Could you check a few things on this model? Use its own coordinates, in mm. A direction names the side the tool comes from. Coordinates: 2 decimals unless noted, no trailing zeros. Loops run counter-clockwise (first coordinate to the right, second up) from the corner with the lowest first, then second, coordinate; pieces in that order, holes last.
from build123d import *

# Parameters (mm, degrees)
BOSS_EXTRUDE1_DEPTH       = 5.842
F_6_32_TAPPED_HOLE1_D     = 2.7051
F_6_32_TAPPED_HOLE1_DEPTH = 0.635
CUT_EXTRUDE1_REACH        = 11.652
SKETCH6_R                 = 2.159
BOSS_EXTRUDE2_DEPTH       = 5.842
CUT_EXTRUDE4_DEPTH        = 10.652


with BuildPart() as part:
    # Sketch1 → Boss-Extrude1 (new body)
    with BuildSketch(Plane.XY):
        Polygon((-3.353873239, 20.18718662), (-3.353873239, -2.29181338), (6.298126761, -2.29181338), (6.298126761, 20.18718662), (5.663126761, 20.18718662), (5.663126761, -1.52981338), (-2.718873239, -1.52981338), (-2.718873239, 20.18718662), align=None)
    extrude(amount=BOSS_EXTRUDE1_DEPTH)

    # #6-32 Tapped Hole1
    with Locations(Plane.ZY.offset(3.353873239)):
        with Locations((2.921, 17.39318662)):
            Hole(F_6_32_TAPPED_HOLE1_D / 2, depth=F_6_32_TAPPED_HOLE1_DEPTH)

    # Sketch6 → Cut-Extrude1 (cut, up to next)
    with BuildSketch(Plane(origin=(6.298126761, 0, 0), x_dir=(0, 0, -1), z_dir=(1, 0, 0)), mode=Mode.PRIVATE) as cut_extrude1_sk1:
        with Locations((-2.921, 17.39318662)):
            Circle(SKETCH6_R)
    cut_extrude1_tool1 = extrude(cut_extrude1_sk1.sketch, amount=-CUT_EXTRUDE1_REACH, mode=Mode.PRIVATE) & part.part
    add(cut_extrude1_tool1.solids().sort_by_distance((6.298127, 17.393187, 2.921))[0], mode=Mode.SUBTRACT)

    # Sketch15 → Boss-Extrude2 (add, through all)
    with BuildSketch(Plane.XY):
        with BuildLine():
            Line((6.298126761, -2.29181338), (-3.353873239, -2.29181338))
            ThreePointArc((-3.353873239, -2.29181338), (1.472126761, -2.477704159), (6.298126761, -2.29181338))
        make_face()
    extrude(amount=BOSS_EXTRUDE2_DEPTH)

    # Sketch28 → Cut-Extrude4 (cut, through all)
    with BuildSketch(Plane(origin=(6.298126761, 0, 0), x_dir=(0, 0, -1), z_dir=(1, 0, 0))):
        with BuildLine():
            Line((-5.842, 20.18718662), (-5.842, 14.860557672))
            add(Edge.make_bspline(
                [(-2.921, 20.18718662), (-5.842, 20.18718662), (-5.842, 14.860557672)],
                knots=[6.283185307, 6.283185307, 6.283185307, 7.853981634, 7.853981634, 7.853981634], degree=2, weights=[1, 0.707106781, 1]))
            Line((-2.920999983, 20.18718662), (-5.842, 20.18718662))
        make_face()
        with BuildLine():
            Line((0, 20.18718662), (-2.920999983, 20.18718662))
            add(Edge.make_bspline(
                [(0, 14.860557672), (0, 20.18718662), (-2.921, 20.18718662)],
                knots=[4.71238898, 4.71238898, 4.71238898, 6.283185307, 6.283185307, 6.283185307], degree=2, weights=[1, 0.707106781, 1]))
            Line((0, 14.860557672), (0, 20.18718662))
        make_face()
    extrude(amount=-CUT_EXTRUDE4_DEPTH, mode=Mode.SUBTRACT)


solid = part.part
(1) Imagine slicing it at D-D, the plane x = -2.5. Write out the boundary of the cut face in (y, z), and give its area (3 significant figures).
Answers:
outline: (-2.35, 0) - (-1.53, 0) - (-1.53, 5.84) - (-2.35, 5.84) - close
area: 4.80 mm2
(2) For pin 1 (3 mm diameter, centred on x = 0.5, z = 3.5, fed in from +Y), with a flat end and sliding along its axis, tell me the tip position at first contact or that it passes through.
Answers:
pin 1: stops at y = -1.53
(3) We'd pull the mould along Y, two halves only. Please class faces 1 (the face through (-3, 4, 0)), 2 (the face through (1.404, -2.478, 2.88)), 3 (the face through (-3.03, 16.19, 2.3)), 4 (the face through (5.985, 15.286, 3.389)): +Y half, -Y half, draft (parallel to the pull), parting line (faces both ways), or undercut.
Answers:
face 1: draft
face 2: -Y half
face 3: undercut
face 4: undercut
(4) Imagine slicing it at A-A, the plane y = -0.25. Write out the boundary of the cut face in (x, z).
Answers:
outline: (-3.35, 0) - (-2.72, 0) - (-2.72, 5.84) - (-3.35, 5.84) - close; (5.66, 0) - (6.3, 0) - (6.3, 5.84) - (5.66, 5.84) - close
(5) Which directions (+Z, -Z, +X, -X, +Y, -Y) give clear straight access to the entire face, cutting with the end or side of a thin tool? Please do faces 5 (the face through (-3.354, 9, 3)), 6 (the face through (-2.719, 9, 3)).
Answers:
face 5: +Z, -Z, -X, +Y, -Y
face 6: +Z, -Z, +Y
(6) Imagine slicing it at B-B, the plane z = 2.35. State how many separate pieces and enclosed holes the cut face has, and give its area (3 significant figures).
Answers:
separate pieces: 3
enclosed holes: 0
area: 31.8 mm2
(7) I need wall thicknesses on probe 1 along X at (y, z) = (11.75, 0.5); probe 2 along Y at (x, z) = (1.5, 3.75); probe 3 along X at (y, z) = (18.75, 4.2). Which ranges of each line are inside material? Lowest first, please.
Answers:
probe 1: x = -3.35 to -2.72, 5.66 to 6.3
probe 2: y = -2.48 to -1.53
probe 3: x = -3.35 to -2.72
